Verification items for the finished model (mm, model axes). Coordinates: 2 decimals unless noted, no trailing zeros. Write each loop counter-clockwise with the first axis right and the second up, starting at its lowest first coordinate (ties: lowest second). Pieces come first, ordered by that corner, then holes. Notation, with made-up numbers: M 53,61 L 64,61 A6 cw 64,71 Z; hole C 13.25,40 d3. An arc over 180 degrees is marked long. One line per item, written item: value.
```python
from build123d import *

# Parameters (mm, degrees)
CROQUIS2_W              = 70
CROQUIS2_H              = 178
SALIENTE_EXTRUIR1_DEPTH = 0.5
SALIENTE_EXTRUIR3_DEPTH = 0.1
CROQUIS7_W              = 22.17688196
CROQUIS7_H              = 3.307809841
CORTAR_EXTRUIR1_DEPTH   = 0.1
CROQUIS12_R             = 0.884703758
CORTAR_EXTRUIR6_DEPTH   = 0.1
SALIENTE_EXTRUIR7_DEPTH = 0.1
CROQUIS14_W             = 28.951405582
CROQUIS14_H             = 2.886934834
CORTAR_EXTRUIR9_DEPTH   = 0.1


with BuildPart() as part:
    # Croquis2 → Saliente-Extruir1 (new body)
    with BuildSketch(Plane.XY):
        Rectangle(CROQUIS2_W, CROQUIS2_H)
    extrude(amount=SALIENTE_EXTRUIR1_DEPTH)

    # Croquis3 → Saliente-Extruir3 (add)
    with BuildSketch(Plane.XY.offset(0.5)):
        with BuildLine():
            Line((-9.855540385, -76.309745211), (10.927527897, -76.309745211))
            ThreePointArc((10.927527897, -76.309745211), (11.793597531, -75.809668594), (11.79346482, -74.809591989))
            Line((11.79346482, -74.809591989), (1.401930679, -56.818279148))
            ThreePointArc((1.401930679, -56.818279148), (0.535993756, -56.31843237), (-0.329943167, -56.818279148))
            Line((-0.329943167, -56.818279148), (-10.721477308, -74.809591989))
            ThreePointArc((-10.721477308, -74.809591989), (-10.721610019, -75.809668594), (-9.855540385, -76.309745211))
        make_face()
    extrude(amount=SALIENTE_EXTRUIR3_DEPTH)

    # Croquis7 → Cortar-Extruir1 (cut)
    with BuildSketch(Plane.XY.offset(0.5)):
        with Locations((0, 81.996928937)):
            Rectangle(CROQUIS7_W, CROQUIS7_H)
    extrude(amount=-CORTAR_EXTRUIR1_DEPTH, mode=Mode.SUBTRACT)

    # Croquis12 → Cortar-Extruir6 (cut)
    with BuildSketch(Plane.XY.offset(0.6)):
        with Locations((0.537972258, -74.332087137)):
            Circle(CROQUIS12_R)
        with BuildLine():
            Line((-0.348710002, -71.972665126), (-1.628640607, -65.425857317))
            ThreePointArc((-1.628640607, -65.425857317), (0.302962598, -63.346803486), (2.382016429, -65.278406691))
            Line((2.382016429, -65.278406691), (1.678502804, -71.951849763))
            ThreePointArc((1.678502804, -71.951849763), (0.674168301, -72.865249783), (-0.348710002, -71.972665126))
        make_face()
    extrude(amount=-CORTAR_EXTRUIR6_DEPTH, mode=Mode.SUBTRACT)

    # Croquis4 → Saliente-Extruir7 (add)
    with BuildSketch(Plane.XY.offset(0.5)):
        Polygon((-4.107800338, -45.327798296), (-7.077418664, -45.327798296), (-10.721484373, -49.854681807), (-7.077418664, -49.854681807), (-11.437215381, -55.270690584), (-12.621463736, -54.317390413), (-12.621463736, -56.74183704), (-9.609666384, -56.74183704), (-10.721484373, -55.846842105), (-3.908016847, -48.520813848), (-7.077418664, -48.520813848), align=None)
        Polygon((9.609666384, -56.74183704), (10.721484373, -55.846842105), (3.908016847, -48.520813848), (7.077418664, -48.520813848), (4.107800338, -45.327798296), (7.077418664, -45.327798296), (10.721484373, -49.854681807), (7.077418664, -49.854681807), (11.437215381, -55.270690584), (12.621463736, -54.317390413), (12.621463736, -56.74183704), align=None)
    extrude(amount=SALIENTE_EXTRUIR7_DEPTH)

    # Croquis14 → Cortar-Extruir9 (cut)
    with BuildSketch(Plane.XY.offset(0.5)):
        with Locations((0, 77.150486091)):
            Rectangle(CROQUIS14_W, CROQUIS14_H)
        with Locations((0, 69.150486091)):
            Rectangle(CROQUIS14_W, CROQUIS14_H)
        with Locations((0, 61.150486091)):
            Rectangle(CROQUIS14_W, CROQUIS14_H)
        with Locations((0, 53.150486091)):
            Rectangle(CROQUIS14_W, CROQUIS14_H)
        with Locations((0, 45.150486091)):
            Rectangle(CROQUIS14_W, CROQUIS14_H)
        with Locations((0, 37.150486091)):
            Rectangle(CROQUIS14_W, CROQUIS14_H)
        with Locations((0, 29.150486091)):
            Rectangle(CROQUIS14_W, CROQUIS14_H)
        with Locations((0, 21.150486091)):
            Rectangle(CROQUIS14_W, CROQUIS14_H)
        with Locations((0, 13.150486091)):
            Rectangle(CROQUIS14_W, CROQUIS14_H)
        with Locations((0, 5.150486091)):
            Rectangle(CROQUIS14_W, CROQUIS14_H)
        with Locations((0, -2.849513909)):
            Rectangle(CROQUIS14_W, CROQUIS14_H)
        with Locations((0, -10.849513909)):
            Rectangle(CROQUIS14_W, CROQUIS14_H)
        with Locations((0, -18.849513909)):
            Rectangle(CROQUIS14_W, CROQUIS14_H)
        with Locations((0, -26.849513909)):
            Rectangle(CROQUIS14_W, CROQUIS14_H)
        with Locations((0, -34.849513909)):
            Rectangle(CROQUIS14_W, CROQUIS14_H)
    extrude(amount=-CORTAR_EXTRUIR9_DEPTH, mode=Mode.SUBTRACT)


solid = part.part
```
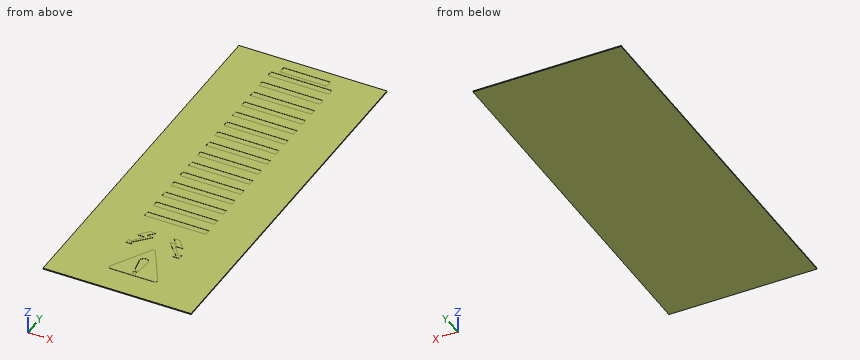
Item 1: Cross-section at A-A, the plane y = -22. Enter the section's corners in (x, z), and give its area (3 significant figures).
The answers:
outline: M -35,0 L 35,0 L 35,0.5 L -35,0.5 Z
area: 35.0 mm²
Item 2: Cross-section at B-B, the plane x = 21. Enter the section's corners in (y, z).
The answers:
outline: M -89,0 L 89,0 L 89,0.5 L -89,0.5 Z
Item 3: Scan lines: line 1 (X direction, y = 81, z = 0.45); line 2 (X direction, y = -55, z = 0.55); line 3 (Z direction, x = 29, y = -39). Record each from-to range of solid material in increasing order.
The answers:
line 1: x = -35 to -11.09, 11.09 to 35
line 2: x = -12.62 to -11.77, -11.22 to -9.93, 9.93 to 11.22, 11.77 to 12.62
line 3: z = 0 to 0.5
